Check sheet for the drawn part. Datum: minimum x, y, z corner. Units: mm. A direction names the side the tool comes from. Coordinates: 2 decimals unless noted, no trailing zeros. Order: outer loops, then holes, each group sorted by start corner. A loop starts at its lowest first (then second) coordinate and runs counter-clockwise, first axis right, second up.
Q1. Depth check by flat-ended pin: P1, Ø1, axis at y = 4.5, z = 1.5, coming from the +X side; P2, Ø3.5, axis at x = 3.75, y = 9.75, coming from the -Z side; P3, Ø6.5, axis at x = 3.5, y = 2, coming from the +Z side; P4, Ø3, axis at x = 3.5, y = 8.5, coming from the -Z side. Enter the tip coordinate at first touch or a pass-through.
Q2. Cross-section at D-D, the plane z = 1.05. Record the boundary of the cut face in (x, y) (3 decimals), and give its area (3 significant figures).
Q3. Thickness scan on line 1 (Y direction, x = 3.5, z = 0.45) (3 decimals); line 2 (X direction, y = 10, z = 1.65) (3 decimals); line 3 (X direction, y = 3, z = 1.5). Record the ranges inside material, lowest first.
Q4. Cross-section at A-A, the plane x = 10.5. Record the boundary of the cut face in (y, z).
Q5. Cross-section at C-C, the plane y = 9.75. Record the boundary of the cut face in (x, z) (3 decimals), and give its area (3 significant figures).
Q6. Cross-section at B-B, the plane z = 2.4. Record the boundary of the cut face in (x, y) (3 decimals), and give its area (3 significant figures).
Q7. Draft check along X on the marked faces 1, 2 and 3. Enter one of: pulls with the +X half, pulls with the -X half, needs draft (parallel to the pull), parting line crosses it, or undercut.
Q8. Set-up check for the marked faces 4, 5, 6, 7 and 8: record each of +Z, -Z, +X, -X, +Y, -Y from which the full face is reachable in a straight line by a thin tool's end or side.
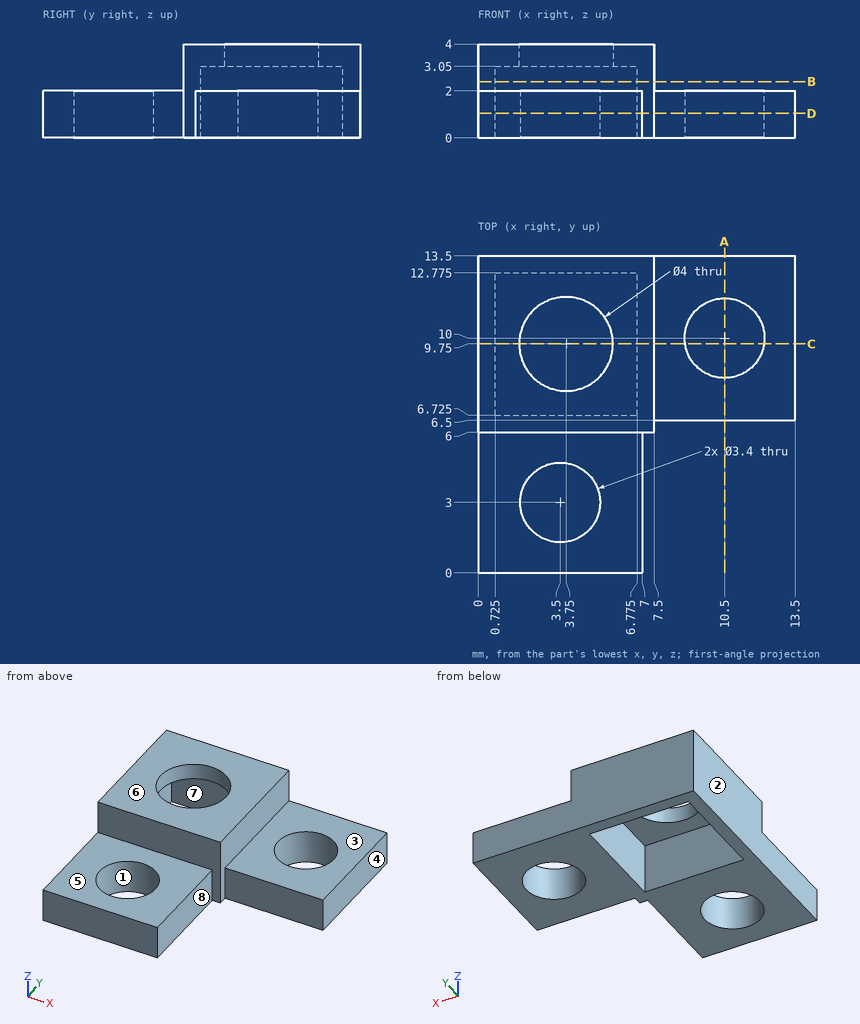
Check values:
1. P1: stops at x = 7
1. P2: passes through
1. P3: stops at z = 2
1. P4: stops at z = 3.05
2. outline: (0, 0) - (7, 0) - (7, 6) - (7.5, 6) - (7.5, 6.5) - (13.5, 6.5) - (13.5, 13.5) - (0, 13.5) - close; hole (0.725, 6.725) - (6.775, 6.725) - (6.775, 12.775) - (0.725, 12.775) - close; hole circle Ø3.4 at (3.5, 3); hole circle Ø3.4 at (10.5, 10)
2. area: 85.5 mm2
3. line 1: y = 0 to 1.3, 4.7 to 6.725, 12.775 to 13.5
3. line 2: x = 0 to 0.725, 6.775 to 8.8, 12.2 to 13.5
3. line 3: x = 0 to 1.8, 5.2 to 7
4. outline: (6.5, 0) - (8.3, 0) - (8.3, 2) - (6.5, 2) - close; (11.7, 0) - (13.5, 0) - (13.5, 2) - (11.7, 2) - close
5. outline: (0, 0) - (0.725, 0) - (0.725, 3.05) - (1.75, 3.05) - (1.75, 4) - (0, 4) - close; (5.75, 3.05) - (6.775, 3.05) - (6.775, 0) - (8.818, 0) - (8.818, 2) - (7.5, 2) - (7.5, 4) - (5.75, 4) - close; (12.182, 0) - (13.5, 0) - (13.5, 2) - (12.182, 2) - close
5. area: 13.0 mm2
6. outline: (0, 6) - (7.5, 6) - (7.5, 13.5) - (0, 13.5) - close; hole (0.725, 6.725) - (6.775, 6.725) - (6.775, 12.775) - (0.725, 12.775) - close
6. area: 19.6 mm2
7. face 1: undercut
7. face 2: pulls with the -X half
7. face 3: needs draft
8. face 4: +Z, -Z, +X, +Y, -Y
8. face 5: +Z, +X, -X, -Y
8. face 6: +Z, +X, -X, +Y, -Y
8. face 7: -Z
8. face 8: +Z, -Z, +X, -Y
